Design review of the part shown in the three views and the two pictorial views. Dimensions are in mm from the part's minimum x, y and z. A direction names the side the tool comes from. Coordinates: 2 decimals unless noted, no trailing zeros. Loops run counter-clockwise (first coordinate to the right, second up) from the corner with the lowest first, then second, coordinate; pieces in that order, holes last. Notation, with made-up numbers: M 65.25,37.25 L 87.25,37.25 A11 cw 87.25,58.25 Z; hole C -25.75,58 d9. An arc over 180 degrees is marked long. Use one line per item in the form item = value.
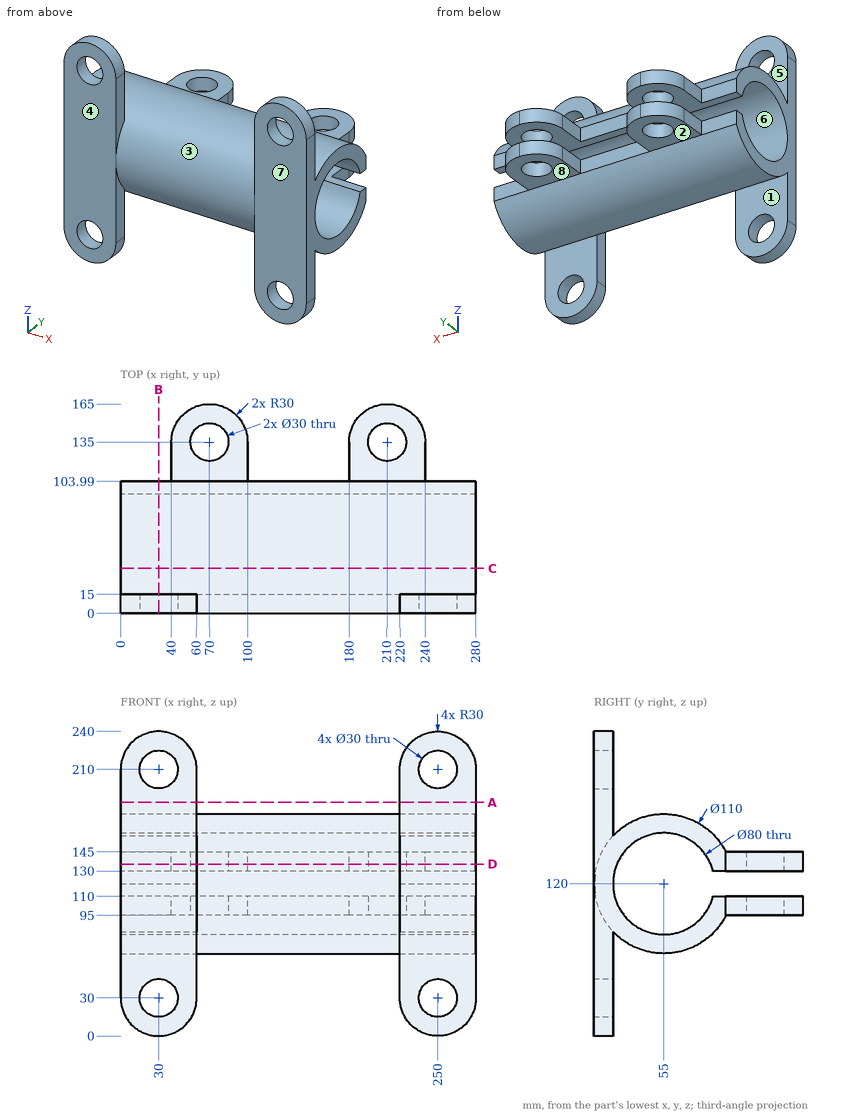
1. Insertion check: P1, Ø18, axis at x = 19.5, z = 199.5, coming from the +Y side; P2, Ø7.5, axis at y = 122, z = 138.5, coming from the -X side; P3, Ø12, axis at x = 256, z = 105, coming from the +Y side. Each pin has a flat end and moves straight along its axis. Give the tip position at first contact, or say it passes through.
Response values:
P1 = 15
P2 = 40
P3 = 103.99
2. Add section C-C (y = 35.5). State the section outline as (x, z) points (1 decimal).
Response values:
outline = M 0,68.6 L 280,68.6 L 280,85.1 L 0,85.1 Z; M 0,154.9 L 280,154.9 L 280,171.4 L 0,171.4 Z
3. Add section D-D (z = 135.5). State the section outline as (x, y) points (1 decimal), then the cut area to 3 significant figures.
Response values:
outline = M 0,0 L 60,0 L 60,2.2 L 220,2.2 L 220,0 L 280,0 L 280,18.1 L 0,18.1 Z; M 0,91.9 L 280,91.9 L 280,104 L 240,104 L 240,135 A30 ccw 180,135 L 180,104 L 100,104 L 100,135 A30 ccw 40,135 L 40,104 L 0,104 Z; hole C 70,135 d30; hole C 210,135 d30
area = 13,200 mm^2
4. The part is to be moulded in two halves that separate along Y. For the marked faces 6, 7 and 8, say which applies: pulls with the +Y half, pulls with the -Y half, needs draft (parallel to the pull), parting line crosses it, or undercut.
Response values:
face_6 = undercut
face_7 = pulls with the -Y half
face_8 = needs draft
5. Add section B-B (x = 30). State the section outline as (y, z) points.
Response values:
outline = M 0,0 L 15,0 L 15,15 L 0,15 Z; M 0,45 L 15,45 L 15,82.25 A55 ccw 103.99,95 L 103.99,110 L 93.73,110 A40 cw long 93.73,130 L 103.99,130 L 103.99,145 A55 ccw 15,157.75 L 15,195 L 0,195 Z; M 0,225 L 15,225 L 15,240 L 0,240 Z
6. Wall thickness on line 1 along Z through (x, y) = (250, 11.25); line 2 along X through (y, z) = (8, 210); line 3 along X through (y, z) = (135, 106): over which ranges is each line inside the solid? List them lowest first. Write a range as from..to.
Response values:
line_1 = 0..15, 45..195, 225..240
line_2 = 0..15, 45..60, 220..235, 265..280
line_3 = 40..55, 85..100, 180..195, 225..240
7. Machinability: for the marked faces 1, 2, 3, 4 and 5, which of the approach directions +Z, -Z, +X, -X, +Y, -Y give a long, thin tool a straight path to every point of the face, cutting with its end or side? Answer none if there is none.
Response values:
face_1 = -Z, +X, -X
face_2 = -Z, +X, -X, +Y
face_3 = none
face_4 = +Z, -Z, +X, -X, -Y
face_5 = +Z, +X, -X
8. Add section A-A (z = 184). State the section outline as (x, y) points, then the cut area to 3 significant figures.
Response values:
outline = M 0,0 L 60,0 L 60,15 L 0,15 Z; M 220,0 L 280,0 L 280,15 L 220,15 Z
area = 1,800 mm^2
